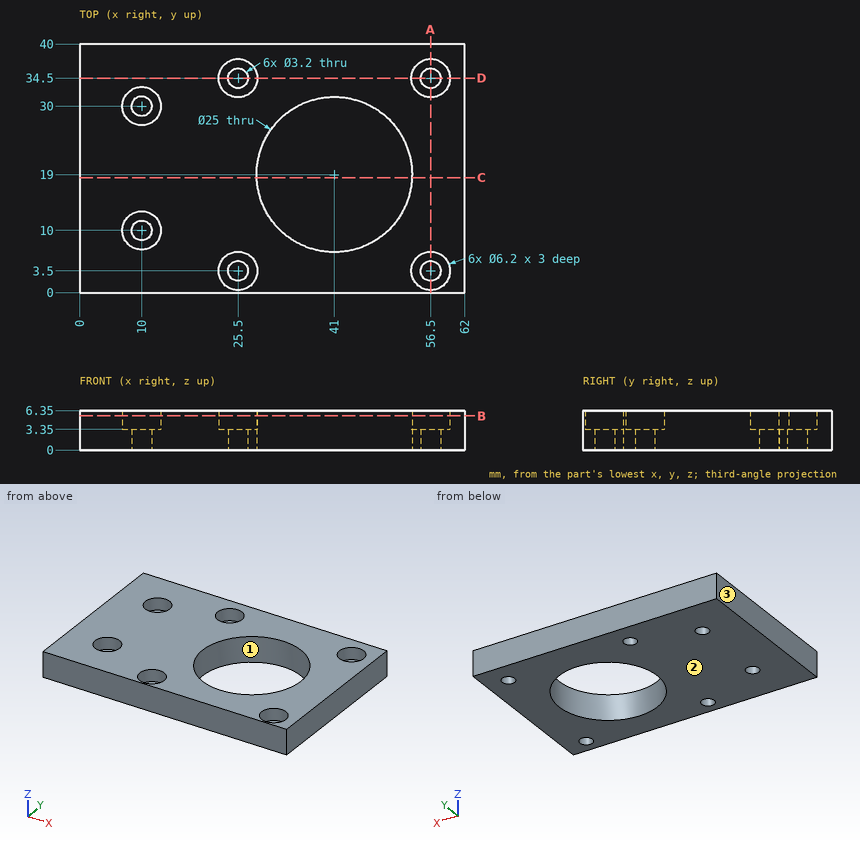
Verification items for this drawing (mm, ordinates from the low corner). Coordinates: 2 decimals unless noted, no trailing zeros. Loops run counter-clockwise (first coordinate to the right, second up) from the corner with the lowest first, then second, coordinate; pieces in that order, holes last. Notation, with made-up numbers: (-3.5, 68) - (5.5, 68) arc R19 ccw to (5.5, 75) - close; hole circle Ø5 at (75, -24.5). An arc over 180 degrees is marked (long way). One line per item, written item: value. Start each with the question number.
(1) Cross-section at C-C on y = 18.5. Enter the section's corners in (x, z), plus the area to 3 significant figures.
(2) Cross-section at D-D on y = 34.5. Enter the section's corners in (x, z), plus the area to 3 significant figures.
(3) Material ranges on line 1 (X direction, y = 34.5, z = 5.5); line 2 (Y direction, x = 25.5, z = 5.05); line 3 (Y direction, x = 10, z = 1.2), recorded low to high. Write a range as [from, to].
(4) Cross-section at A-A on x = 56.5. Enter the section's corners in (y, z), plus the area to 3 significant figures.
(5) Depth check by flat-ended pin: P1, Ø3.5, axis at x = 56.5, y = 3.5, coming from the +Z side. Enter the tip coordinate at first touch or a pass-through.
(6) Cross-section at B-B on z = 5.5. Enter the section's corners in (x, y), plus the area to 3 significant figures.
(7) Mould release check, pull along X, two halves, no side actions. Record for the marked faces 1, 2 and 3: released by +X, released by -X, zero draft, split by the parting line, or undercut.
Results below:
1. outline: (0, 0) - (28.51, 0) - (28.51, 6.35) - (0, 6.35) - close; (53.49, 0) - (62, 0) - (62, 6.35) - (53.49, 6.35) - close
1. area: 235 mm2
2. outline: (0, 0) - (23.9, 0) - (23.9, 3.35) - (22.4, 3.35) - (22.4, 6.35) - (0, 6.35) - close; (27.1, 0) - (54.9, 0) - (54.9, 3.35) - (53.4, 3.35) - (53.4, 6.35) - (28.6, 6.35) - (28.6, 3.35) - (27.1, 3.35) - close; (58.1, 0) - (62, 0) - (62, 6.35) - (59.6, 6.35) - (59.6, 3.35) - (58.1, 3.35) - close
2. area: 335 mm2
3. line 1: x = [0, 22.4], [28.6, 53.4], [59.6, 62]
3. line 2: y = [0, 0.4], [6.6, 31.4], [37.6, 40]
3. line 3: y = [0, 8.4], [11.6, 28.4], [31.6, 40]
4. outline: (0, 0) - (1.9, 0) - (1.9, 3.35) - (0.4, 3.35) - (0.4, 6.35) - (0, 6.35) - close; (5.1, 0) - (32.9, 0) - (32.9, 3.35) - (31.4, 3.35) - (31.4, 6.35) - (6.6, 6.35) - (6.6, 3.35) - (5.1, 3.35) - close; (36.1, 0) - (40, 0) - (40, 6.35) - (37.6, 6.35) - (37.6, 3.35) - (36.1, 3.35) - close
4. area: 195 mm2
5. P1: stops at z = 3.35
6. outline: (0, 0) - (62, 0) - (62, 40) - (0, 40) - close; hole circle Ø6.2 at (10, 10); hole circle Ø6.2 at (10, 30); hole circle Ø6.2 at (25.5, 3.5); hole circle Ø6.2 at (25.5, 34.5); hole circle Ø25 at (41, 19); hole circle Ø6.2 at (56.5, 3.5); hole circle Ø6.2 at (56.5, 34.5)
6. area: 1,810 mm2
7. face 1: undercut
7. face 2: zero draft
7. face 3: released by -X
